Autodesk Inventor part; units mm, degrees
ref_plane "YZ Plane" through (0, 0, 0) normal (1, 0, 0) x (0, 1, 0)
ref_plane "XZ Plane" through (0, 0, 0) normal (0, 1, 0) x (-1, 0, 0)
ref_plane "XY Plane" through (0, 0, 0) normal (0, 0, 1) x (1, 0, 0)
sketch "Sketch1" plane through (0, 0, 0) normal (0, 1, 0) x (-1, 0, 0)
  point P0 (0, 0)
sketch "Sketch2" plane through (0, 0, 0) normal (0, 1, 0) x (-1, 0, 0)
  line L0 (0, 0) -> (-31, 0)
  line L1 (-31, -1.65) -> (-31, -29.35)
  line L2 (-31, -31) -> (0, -31)
  line L3 (0, -29.35) -> (0, -1.65)
  circle A0 centre (0, 0) radius 1.65
  circle A1 centre (0, -31) radius 1.65
  circle A2 centre (-31, -31) radius 1.65
  circle A3 centre (-31, 0) radius 1.65
  line L4 (-15.5, -15.5) -> (-15.5, -45.5)
  line L5 (-15.5, 0) -> (-15.5, 14.5)
  circle A4 centre (-15.5, 14.5) radius 2.65
  circle A5 centre (-15.5, -45.5) radius 2.65
  line L6 (9.5, 34.5) -> (-40.5, 34.5)
  line L7 (-40.5, 34.5) -> (-40.5, -65.5)
  line L8 (-40.5, -65.5) -> (9.5, -65.5)
  line L9 (9.5, -65.5) -> (9.5, 34.5)
  line L10 (9.5, 34.5) -> (-40.5, -65.5) construction
  line L11 (-40.5, 34.5) -> (9.5, -65.5) construction
  line L12 (-8, -8) -> (-23, -8)
  line L13 (-23, -8) -> (-23, -23)
  line L14 (-23, -23) -> (-8, -23)
  line L15 (-8, -23) -> (-8, -8)
  line L16 (-8, -8) -> (-23, -23) construction
  line L17 (-23, -8) -> (-8, -23) construction
  dimension "d2" = 3.3
  dimension "d3" = 3.3
  dimension "d4" = 3.3
  dimension "d5" = 3.3
  dimension "d0" = 31
  dimension "d1" = 31
  dimension "d6" = 30
  dimension "d7" = 30
  dimension "d8" = 5.3
  dimension "d9" = 5.3
  dimension "d10" = 50
  dimension "d11" = 100
  dimension "d12" = 15
  dimension "d13" = 15
extrude "Extrusion1" add sketch "Sketch2" along normal blind 5 contours L0 A0 L3 A1 L2 A2 L1 A3 | L9 L8 L7 L6
chamfer "Chamfer1" distance 2 angle 45 8 edges at (40.5, 2.5, 34.5) (40.5, 2.5, -65.5) (-9.5, 2.5, -65.5) (-9.5, 2.5, 34.5) (40.5, 5, -15.5) (15.5, 5, -65.5) (-9.5, 5, -15.5) (15.5, 5, 34.5)
properties part number "nema y axis cover"
Input: part model. Units: mm. Frame: model coordinates. A direction names the side the tool comes from. Round coordinates to 2 decimals unless told otherwise and drop trailing zeros. Order: outer loops, then holes, each group sorted by start corner. A loop starts at its lowest first (then second) coordinate and runs counter-clockwise, first axis right, second up.
1. Cut plane A-A, the plane x = 0. Output: boundary loops of the cut face in (y, z), then the cut area to 3 significant figures.
The answers:
outline: (0, -65.5) - (3, -65.5) - (5, -63.5) - (5, -32.65) - (0, -32.65) - close; (0, -29.35) - (5, -29.35) - (5, -1.65) - (0, -1.65) - close; (0, 1.65) - (5, 1.65) - (5, 32.5) - (3, 34.5) - (0, 34.5) - close
area: 463 mm2
2. Cut plane D-D, the plane z = 0. Output: boundary loops of the cut face in (x, y), then the cut area to 3 significant figures.
The answers:
outline: (-9.5, 0) - (-1.65, 0) - (-1.65, 5) - (-7.5, 5) - (-9.5, 3) - close; (1.65, 0) - (29.35, 0) - (29.35, 5) - (1.65, 5) - close; (32.65, 0) - (40.5, 0) - (40.5, 3) - (38.5, 5) - (32.65, 5) - close
area: 213 mm2
3. Set-up query: faces 5 (the face through (15, 2, -8)), 6 (the face through (-8, 4, 33)). Return all of +Z, -Z, +X, -X, +Y, -Y with unobstructed straight access to the full face (end or side cutting, diameter ignored); none if empty.
The answers:
face 5: +Y, -Y
face 6: +Z, -X, +Y
4. Cut plane B-B, the plane z = -45.5. Output: boundary loops of the cut face in (x, y).
The answers:
outline: (-9.5, 0) - (12.85, 0) - (12.85, 5) - (-7.5, 5) - (-9.5, 3) - close; (18.15, 0) - (40.5, 0) - (40.5, 3) - (38.5, 5) - (18.15, 5) - close
5. Material intervals for line 1 (Z direction, x = 31, y = 2.7); line 2 (X direction, y = 1.2, z = 0); line 3 (Z direction, x = 15.5, y = 2.85), sorted ascending.
The answers:
line 1: z = -65.5 to -32.65, -29.35 to -1.65, 1.65 to 34.5
line 2: x = -9.5 to -1.65, 1.65 to 29.35, 32.65 to 40.5
line 3: z = -65.5 to -48.15, -42.85 to -23, -8 to 11.85, 17.15 to 34.5
6. Cut plane C-C, the plane y = 1.05. Output: boundary loops of the cut face in (x, z).
The answers:
outline: (-9.5, -63.5) - (-7.5, -65.5) - (38.5, -65.5) - (40.5, -63.5) - (40.5, 32.5) - (38.5, 34.5) - (-7.5, 34.5) - (-9.5, 32.5) - close; hole circle Ø3.3 at (0, -31); hole circle Ø3.3 at (0, 0); hole (8, -23) - (23, -23) - (23, -8) - (8, -8) - close; hole circle Ø5.3 at (15.5, -45.5); hole circle Ø5.3 at (15.5, 14.5); hole circle Ø3.3 at (31, -31); hole circle Ø3.3 at (31, 0)
7. Mould query, pull axis X, two halves, no side actions, for faces 1 (the face through (39, 4, -64)), 2 (the face through (8, 2, -16)), 3 (the face through (31.215, 2.465, -32.636)), 4 (the face through (16, 0, -4)). Classes: released by +X, released by -X, zero draft, split by the parting line, or undercut.
The answers:
face 1: released by +X
face 2: undercut
face 3: undercut
face 4: zero draft
